Can you work these out from the model? Positions are in its coordinate system, mm. A direction names the side the tool comes from. Coordinates: 2 decimals unless noted, no trailing zeros. Order: outer loops, then holes, each group sorted by start corner. A loop starts at its lowest first (then second) coordinate and runs counter-clockwise, first axis right, second up. Notation, with made-up numbers: (-17, 32) - (31, 32) arc R15 ccw to (31, 42) - close; hole circle Ø7 at (-40, 73.5). An arc over 180 degrees is marked (long way). Return JSON: item names as keys, results as strings. Group by question number.
1) Imagine slicing it at A-A (z = 5.5). Write out the boundary of the cut face in (x, y), and give its area (3 significant figures).
2) For pin 1 Ø15 at (x, z) = (-2.5, 4.5) entering from +Y, with a flat end and sliding along its axis, tell me the tip position at first contact or that it passes through.
3) If we mould it in two halves opening along X, with no side actions, what happens to faces 3 (the face through (-15, 1, 0)), 4 (the face through (15, 1, 0)), 5 (the face through (0, 1, -15)), 6 (the face through (0.14, 0.7, -9.43))? For each: pulls with the +X half, pulls with the -X half, needs draft (parallel to the pull), parting line crosses it, or undercut.
4) Imagine slicing it at D-D (x = -12.5). Write out the boundary of the cut face in (y, z), and give its area (3 significant figures).
5) Imagine slicing it at B-B (x = -4). Write out the boundary of the cut face in (y, z), and give its area (3 significant figures).
6) If I drill on line 1 along Z through (x, y) = (-5, 2.4); line 2 along Y through (x, z) = (3.25, -11); line 3 along Z through (x, y) = (7.25, 1.6), over which ranges is the centre line in solid material (lowest first)?
7) Imagine slicing it at C-C (y = 3.5). Write out the boundary of the cut face in (x, z), and give its area (3 significant figures).
8) Which directions (+Z, -Z, +X, -X, +Y, -Y) give clear straight access to the entire face, cutting with the end or side of a thin tool? Please do faces 1 (the face through (9.43, 0.7, -0.14)), 2 (the face through (12, 5, -13)).
```python
from build123d import *

# Parameters (mm, degrees)
SKETCH1_W           = 20
SKETCH1_H           = 20
SKETCH1_W_2         = 15
SKETCH1_H_2         = 15
BOSS_EXTRUDE3_DEPTH = 0.1
SKETCH1_5_W         = 30
SKETCH1_5_H         = 30
SKETCH1_5_W_2       = 20
SKETCH1_5_H_2       = 20
BOSS_EXTRUDE4_DEPTH = 2.5
FILLET2_R           = 2
BOSS_EXTRUDE5_DEPTH = 2.5


with BuildPart() as part:
    # Sketch1 → Boss-Extrude3 (new body)
    with BuildSketch(Plane(origin=(0, 0, 0), x_dir=(1, 0, 0), z_dir=(0, 1, 0))):
        Rectangle(SKETCH1_W, SKETCH1_H)
        Rectangle(SKETCH1_W_2, SKETCH1_H_2, mode=Mode.SUBTRACT)
    extrude(amount=BOSS_EXTRUDE3_DEPTH)

    # Sketch1_5 → Boss-Extrude4 (add)
    with BuildSketch(Plane(origin=(0, 0, 0), x_dir=(1, 0, 0), z_dir=(0, 1, 0))):
        Rectangle(SKETCH1_5_W, SKETCH1_5_H)
        Rectangle(SKETCH1_5_W_2, SKETCH1_5_H_2, mode=Mode.SUBTRACT)
    extrude(amount=BOSS_EXTRUDE4_DEPTH)

    # Fillet2
    fillet2_edges = [part.edges().sort_by_distance(p)[0] for p in [
        (0, 0.1, 10),
        (10, 0.1, 0),
        (0, 0.1, -10),
        (-10, 0.1, 0),
    ]]
    fillet(fillet2_edges, radius=FILLET2_R)

    # Sketch2 → Boss-Extrude5 (add)
    with BuildSketch(Plane(origin=(0, 2.5, 0), x_dir=(1, 0, 0), z_dir=(0, 1, 0))):
        with BuildLine():
            ThreePointArc((14, -12.5), (13.074025149, -11.114180701), (11.439339828, -11.439339828))
            Line((11.439339828, -11.439339828), (13.560660172, -13.560660172))
            ThreePointArc((13.560660172, -13.560660172), (13.885819299, -13.074025149), (14, -12.5))
        make_face()
        with BuildLine():
            Line((13.560660172, -13.560660172), (11.439339828, -11.439339828))
            ThreePointArc((11.439339828, -11.439339828), (11.439339828, -13.560660172), (13.560660172, -13.560660172))
        make_face()
        with BuildLine():
            ThreePointArc((14, 12.5), (13.885819299, 13.074025149), (13.560660172, 13.560660172))
            Line((13.560660172, 13.560660172), (11.439339828, 11.439339828))
            ThreePointArc((11.439339828, 11.439339828), (13.074025149, 11.114180701), (14, 12.5))
        make_face()
        with BuildLine():
            Line((11.439339828, 11.439339828), (13.560660172, 13.560660172))
            ThreePointArc((13.560660172, 13.560660172), (11.439339828, 13.560660172), (11.439339828, 11.439339828))
        make_face()
        with BuildLine():
            ThreePointArc((-11, 12.5), (-11.925974851, 13.885819299), (-13.560660172, 13.560660172))
            Line((-13.560660172, 13.560660172), (-11.439339828, 11.439339828))
            ThreePointArc((-11.439339828, 11.439339828), (-11.114180701, 11.925974851), (-11, 12.5))
        make_face()
        with BuildLine():
            Line((-11.439339828, 11.439339828), (-13.560660172, 13.560660172))
            ThreePointArc((-13.560660172, 13.560660172), (-13.560660172, 11.439339828), (-11.439339828, 11.439339828))
        make_face()
        with BuildLine():
            ThreePointArc((-11, -12.5), (-11.114180701, -11.925974851), (-11.439339828, -11.439339828))
            Line((-11.439339828, -11.439339828), (-13.560660172, -13.560660172))
            ThreePointArc((-13.560660172, -13.560660172), (-11.925974851, -13.885819299), (-11, -12.5))
        make_face()
        with BuildLine():
            Line((-13.560660172, -13.560660172), (-11.439339828, -11.439339828))
            ThreePointArc((-11.439339828, -11.439339828), (-13.560660172, -11.439339828), (-13.560660172, -13.560660172))
        make_face()
    extrude(amount=BOSS_EXTRUDE5_DEPTH)


solid = part.part
```
Calculated:
{
 "1": {"outline": "(-15, 0) - (-7.5, 0) - (-7.5, 0.1) - (-8, 0.1) arc R2 cw to (-10, 2.1) - (-10, 2.5) - (-15, 2.5) - close; (7.5, 0) - (15, 0) - (15, 2.5) - (10, 2.5) - (10, 2.1) arc R2 cw to (8, 0.1) - (7.5, 0.1) - close", "area": "27.2 mm2"},
 "2": {"pin 1": "y = 2.5"},
 "3": {"face 3": "pulls with the -X half", "face 4": "pulls with the +X half", "face 5": "needs draft", "face 6": "undercut"},
 "4": {"outline": "(0, -15) - (2.5, -15) - (2.5, -14) - (5, -14) - (5, -11) - (2.5, -11) - (2.5, 11) - (5, 11) - (5, 14) - (2.5, 14) - (2.5, 15) - (0, 15) - close", "area": "90.0 mm2"},
 "5": {"outline": "(0, -15) - (2.5, -15) - (2.5, -10) - (2.1, -10) arc R2 cw to (0.1, -8) - (0.1, -7.5) - (0, -7.5) - close; (0, 7.5) - (0.1, 7.5) - (0.1, 8) arc R2 cw to (2.1, 10) - (2.5, 10) - (2.5, 15) - (0, 15) - close", "area": "27.2 mm2"},
 "6": {"line 1": "-15 to -10, 10 to 15", "line 2": "0 to 2.5", "line 3": "-15 to -9.94, 9.94 to 15"},
 "7": {"outline": "circle Ø3 at (-12.5, -12.5); circle Ø3 at (-12.5, 12.5); circle Ø3 at (12.5, -12.5); circle Ø3 at (12.5, 12.5)", "area": "28.3 mm2"},
 "8": {"face 1": "+Y", "face 2": "+Z, -Z, +X, -X, +Y"}
}
